Build history of the part. All positions in model axes, mm. A direction names the side the tool comes from. Give positions to 0.01 mm unless a question says otherwise; leave off trailing zeros. Loops run counter-clockwise (first coordinate to the right, second up) from the corner with the lowest first, then second, coordinate; pieces in that order, holes last. Notation, with made-up numbers: M 75.5,-36 L 115.5,-36 A9 cw 115.5,-26 Z; hole C 24.5,-27.75 d6. An arc over 180 degrees is marked long. Answer in a Markdown table with one row per item. Add a question column.
```python
from build123d import *


with BuildPart() as part:
    # Sketch1 → Revolve1 (revolve)
    with BuildSketch(Plane.XY, mode=Mode.PRIVATE) as revolve1_sk:
        Polygon((-38.4, 0), (-38.4, 13.5), (-34.4, 13.5), (-34.4, 15.354591962), (-34.287468985, 15.5), (-22.895018976, 15.5), (-22.895018976, 15.246920735), (-22.595018976, 15.246920735), (-22.595018976, 15.5), (-18.123640766, 15.5), (-18.123640766, 15.246920735), (-17.823640766, 15.246920735), (-17.823640766, 15.5), (-12.771458761, 15.5), (-12.771458761, 14.899770288), (-12.471458761, 14.899770288), (-12.471458761, 15), (-8.004107003, 15), (-7.9, 14.660301421), (-7.9, 12.7), (-3.799837925, 12.7), (-3.799837925, 7.515096405), (-3.499837925, 7.515096405), (-3.499837925, 8), (-0.240891884, 8), (0, 7.777504369), (0, 0), align=None)
    revolve(revolve1_sk.sketch.rotate(Axis((-61.595871807, 0, 0), (1, 0, 0)), 90), axis=Axis((-61.595871807, 0, 0), (1, 0, 0)))

    # Sketch2 → Revolve2 (revolve)
    with BuildSketch(Plane(origin=(0, 0, 0), x_dir=(1, 0, 0), z_dir=(0, 1, 0))):
        with BuildLine():
            Line((-38.4, -9.112860892), (-38.4, 0))
            Line((-38.4, 0), (-40.611277306, 0))
            ThreePointArc((-40.611277306, 0), (-40.124324385, -4.706557364), (-38.4, -9.112860892))
        make_face()
    revolve(axis=Axis((-49.369562138, 0, 0), (1, 0, 0)))


solid = part.part
```
(1) Pin check, flat tips, straight feed: pin 1 (2 mm diameter, centred on x = -11, y = -1.5, fed in from -Z); pin 2 (1 mm diameter, centred on y = -7.5, z = 1.5, fed in from -X); pin 3 (2 mm diameter, centred on x = -27.5, z = 5, fed in from +Y) (3 decimals); pin 4 (9 mm diameter, centred on y = 5.5, z = 4.5, fed in from +X). Stop position of each tip, or through.
(2) Slice it at B-B, the plane x = -29.5. Give the cut face in (y, z).
(3) Pull direction X, two halves, no side cores. Call faces 1 (the flat face through (-3.5, 6, -5)), 2 (the cylindrical face through (-1.85, 7.81, -1.73)), 3 (the flat face through (-7.9, -7, -11)): +X half, -X half, draft (parallel to the pull), parting line (faces both ways), or undercut.
(4) Wall check: line 1 (X direction, y = 9.5, z = 6.5); line 2 (X direction, y = -3, z = 14); line 3 (Y direction, x = -7.5, z = 0). Give the ranges that are in metal, low to high.
(5) Slice it at A-A, the plane x = -5. Give the cut face in (y, z), then the cut area to 3 significant figures.
(6) Tool access for faces 4 (the cylindrical face through (-5.8, 7.7, -10.1)), 5 (the cylindrical face through (-20.328, -15.368, -2.018)), 6 (the cylindrical face through (-36.37, 13.18, -2.93)): list every direction of +Z, -Z, +X, -X, +Y, -Y with a clear straight run to the whole face (end or side of a thin tool).
Solution:
| question | item | result |
|---|---|---|
| 1 | pin 1 | z = -14.99 |
| 1 | pin 2 | x = -39.34 |
| 1 | pin 3 | y = 14.975 |
| 1 | pin 4 | x = 0 |
| 2 | outline | C 0,0 d31 |
| 3 | face 1 | undercut |
| 3 | face 2 | draft |
| 3 | face 3 | +X half |
| 4 | line 1 | -38.4 to -3.8 |
| 4 | line 2 | -34.4 to -7.9 |
| 4 | line 3 | -12.7 to 12.7 |
| 5 | outline | C 0,0 d25.4 |
| 5 | area | 507 mm^2 |
| 6 | face 4 | +X |
| 6 | face 5 | +X, -X |
| 6 | face 6 | -X |
